Model file for the job. Use its own axes, mm. A direction names the side the tool comes from. Round coordinates to 2 decimals unless told otherwise and drop trailing zeros. Order: outer loops, then holes, each group sorted by start corner. A loop starts at its lowest first (then second) coordinate and runs counter-clockwise, first axis right, second up. Notation, with made-up numbers: (-38, -21.5) - (-27, -21.5) arc R17 cw to (-27, 5.5) - close; hole circle Ø3 at (17, 88.5). An arc over 180 degrees is marked (long way). Put each result on its own line as item: value. Start each with the question number.
Item 1: Saw through at A-A on z = 16.5. List the corners of the cut face in (x, y).
Item 2: Pin check, flat tips, straight feed: pin 1 Ø1 at (x, y) = (28.5, 58) entering from +Z; pin 2 Ø2 at (x, y) = (8.5, 40) entering from -Z; pin 3 Ø8 at (x, y) = (20, 41.5) entering from +Z; pin 4 Ø2 at (x, z) = (49.5, 6) entering from +Y. Stop position of each tip, or through.
Item 3: Which spindle directions (+Z, -Z, +X, -X, +Y, -Y) get a long thin tool onto all of the face, cutting with end or side? Do faces 4 (the face through (39, 30, 0)), 5 (the face through (40, 58, 4)), 6 (the face through (40, 3.33, 3)), 7 (the face through (77, 5, 19)), 8 (the face through (3, 58, 34)). Say none if no direction does.
Item 4: Mould opens along X. For faces 1 (the face through (3, 5, 19)), 2 (the face through (40, 30, 2)), 3 (the face through (80, 30, 3)) say: pulls with the +X half, pulls with the -X half, needs draft (parallel to the pull), parting line crosses it, or undercut.
Item 5: Probe probe 1 along X at (y, z) = (58, 5.5); probe 2 along Z at (x, y) = (76, 15); probe 3 along Z at (x, y) = (27, 19.5). List the from-to ranges inside material, lowest first.
Item 6: Saw through at C-C on y = 17.5. List the corners of the cut face in (x, z), plus the area to 3 significant figures.
Item 7: Saw through at B-B on x = 75.5. List the corners of the cut face in (y, z), plus the area to 3 significant figures.
Autodesk Inventor part; units mm, degrees
ref_plane "YZ Plane" through (0, 0, 0) normal (1, 0, 0) x (0, 1, 0)
ref_plane "XZ Plane" through (0, 0, 0) normal (0, 1, 0) x (-1, 0, 0)
ref_plane "XY Plane" through (0, 0, 0) normal (0, 0, 1) x (1, 0, 0)
sketch "Эскиз1" plane through (0, 0, 0) normal (0, 0, 1) x (1, 0, 0)
  line L0 (0, 0) -> (80, 0)
  line L1 (80, 0) -> (80, 60)
  line L2 (80, 60) -> (0, 60)
  line L3 (0, 60) -> (0, 0)
  dimension "d0" = 60
  dimension "d1" = 80
extrude "Выдавливание1" add sketch "Эскиз1" along normal blind 4
ref_plane "РабПлоскость1" through (0, 0, 4) normal (0, 0, 1) x (1, 0, 0)
sketch "Эскиз3" plane through (0, 0, 4) normal (0, 0, 1) x (1, 0, 0)
  line L0 (5.5, 56.67) -> (74.5, 56.67)
  line L1 (74.5, 56.67) -> (74.5, 3.33)
  line L2 (74.5, 3.33) -> (5.5, 3.33)
  line L3 (5.5, 3.33) -> (5.5, 56.67)
  line L4 (80, 60) -> (0, 60)
  line L5 (80, 0) -> (80, 60)
  line L6 (0, 0) -> (80, 0)
  dimension "d5" = 69
  dimension "d6" = 53.34
  dimension "d7" = 3.33
  dimension "d8" = 5.5
  dimension "d11" = 60
  dimension "d12" = 80
extrude "Выдавливание2" cut sketch "Эскиз3" against normal blind 2
sketch "Эскиз4" plane through (0, 0, 4) normal (0, 0, 1) x (1, 0, 0)
  line L0 (80, 60) -> (0, 60)
  line L1 (0, 60) -> (0, 0)
  line L2 (5.5, 56.67) -> (74.5, 56.67)
  line L3 (5.5, 3.33) -> (5.5, 56.67)
  line L4 (80, 0) -> (80, 60)
  line L5 (74.5, 56.67) -> (74.5, 3.33)
  line L6 (74.5, 3.33) -> (5.5, 3.33)
  line L7 (0, 0) -> (80, 0)
  line L8 (5.5, 3.33) -> (5.5, 56.67)
  line L9 (0, 60) -> (5.5, 60)
  line L10 (5.5, 60) -> (5.5, 55)
  line L11 (5.5, 55) -> (0, 55)
  line L12 (0, 55) -> (0, 60)
  line L13 (80, 60) -> (0, 60)
  line L14 (74.5, 56.67) -> (74.5, 3.33)
  line L15 (80, 60) -> (74.5, 60)
  line L16 (74.5, 60) -> (74.5, 55)
  line L17 (74.5, 55) -> (80, 55)
  line L18 (80, 55) -> (80, 60)
  line L19 (80, 0) -> (74.5, 0)
  line L20 (74.5, 0) -> (74.5, 5)
  line L21 (74.5, 5) -> (80, 5)
  line L22 (80, 5) -> (80, 0)
  line L23 (0, 0) -> (5.5, 0)
  line L24 (5.5, 0) -> (5.5, 5)
  line L25 (5.5, 5) -> (0, 5)
  line L26 (0, 5) -> (0, 0)
  dimension "d13" = 5
  dimension "d14" = 5
  dimension "d15" = 5
extrude "Выдавливание3" add sketch "Эскиз4" along normal blind 30 contours L4 L17 L5 L16 L0 | L10 L3 L11 L1 L0 | L4 L7 L20 L5 L21 | L25 L3 L24 L7 L1
equation "\"d7\" = -0.5 * d6 + 0.5 * d11"
equation "\"d8\" = -0.5 * d5 + 0.5 * d12"
properties part number "Каркас для плат"
Results found:
1. outline: (0, 0) - (5.5, 0) - (5.5, 5) - (0, 5) - close; (0, 55) - (5.5, 55) - (5.5, 60) - (0, 60) - close; (74.5, 0) - (80, 0) - (80, 5) - (74.5, 5) - close; (74.5, 55) - (80, 55) - (80, 60) - (74.5, 60) - close
2. pin 1: stops at z = 4
2. pin 2: stops at z = 0
2. pin 3: stops at z = 2
2. pin 4: passes through
3. face 4: -Z, +X, -X, +Y, -Y
3. face 5: +Z, +Y, -Y
3. face 6: +Z
3. face 7: +Z, +X, -X
3. face 8: +Z, +X, -X, +Y, -Y
4. face 1: needs draft
4. face 2: undercut
4. face 3: pulls with the +X half
5. probe 1: x = 0 to 5.5, 74.5 to 80
5. probe 2: z = 0 to 4
5. probe 3: z = 0 to 2
6. outline: (0, 0) - (80, 0) - (80, 4) - (74.5, 4) - (74.5, 2) - (5.5, 2) - (5.5, 4) - (0, 4) - close
6. area: 182 mm²
7. outline: (0, 0) - (60, 0) - (60, 34) - (55, 34) - (55, 4) - (5, 4) - (5, 34) - (0, 34) - close
7. area: 540 mm²
